from build123d import *

# Parameters (mm, degrees)
SKETCH_1_W          = 32
SKETCH_1_H          = 24
EXTRUDE_1_DEPTH     = 20
EXTRUDE_2_DEPTH     = 0.6
SKETCH_3_R          = 1.75
CUT_EXTRUDE_1_DEPTH = 34.111327367
FILLET_1_R          = 3
SKETCH_4_R          = 1.241957667
SKETCH_4_R_2        = 1.176925768
EXTRUDE_3_DEPTH     = 10
SKETCH_5_R          = 1.255951998
SKETCH_5_R_2        = 1.449746198
EXTRUDE_4_DEPTH     = 15


with BuildPart() as part:
    # 草图1 → 凸台-拉伸1 (new body)
    with BuildSketch(Plane.XY):
        Rectangle(SKETCH_1_W, SKETCH_1_H)
    extrude(amount=EXTRUDE_1_DEPTH)

    # 草图2 → 凸台-拉伸2 (add)
    with BuildSketch(Plane.XY):
        Polygon((-16, 12), (-24, 0), (-16, -12), align=None)
        Polygon((16, -12), (16, 12), (24, 0), align=None)
    extrude(amount=EXTRUDE_2_DEPTH)

    # 草图3 → 切除-拉伸1 (cut, through all)
    with BuildSketch(Plane.XY.offset(0.6)):
        with Locations((-20, 0)):
            Circle(SKETCH_3_R)
        with Locations((20, 0)):
            Circle(SKETCH_3_R)
    extrude(amount=-CUT_EXTRUDE_1_DEPTH, mode=Mode.SUBTRACT)

    # 圆角1
    fillet_1_edges = [part.edges().sort_by_distance(p)[0] for p in [
        (24, 0, 0.3),
        (-24, 0, 0.3),
    ]]
    fillet(fillet_1_edges, radius=FILLET_1_R)

    # 草图4 → 凸台-拉伸3 (add)
    with BuildSketch(Plane(origin=(0, 12, 0), x_dir=(1, 0, 0), z_dir=(0, 1, 0))):
        with Locations(Location((-8.72556125, -5.075346112, 0), (0, 0, 90))):
            Circle(SKETCH_4_R)
        with Locations(Location((7.271301042, -5.075346112, 0), (0, 0, 90))):
            Circle(SKETCH_4_R_2)
    extrude(amount=EXTRUDE_3_DEPTH)

    # 草图5 → 凸台-拉伸4 (add)
    with BuildSketch(Plane.XZ.offset(12)):
        with Locations(Location((-10.840848826, 6.265195374, 0), (0, 0, 90))):
            Circle(SKETCH_5_R)
        with Locations(Location((-0.462719157, 6.265195374, 0), (0, 0, 90))):
            Circle(SKETCH_5_R)
        with Locations(Location((7.932328409, 6.265195374, 0), (0, 0, 90))):
            Circle(SKETCH_5_R_2)
    extrude(amount=EXTRUDE_4_DEPTH)


solid = part.part
Design review of the part built by this model. Coordinates are the model's own, in mm. A direction names the side the tool comes from. Coordinates: 2 decimals unless noted, no trailing zeros. Write each loop counter-clockwise with the first axis right and the second up, starting at its lowest first coordinate (ties: lowest second). Pieces come first, ordered by that corner, then holes. Notation, with made-up numbers: (76, -27) -> (115, -27) arc R15 ccw to (115, 0) -> close; hole circle Ø5 at (-22.75, 78). An arc over 180 degrees is marked (long way). Write each question's results on one line, items separated by ' | '. Start each with the question number.
(1) Tool access review of faces 1 (the face through (-7.97, 16.93, 6.06)), 2 (the face through (8, -27, 6)), 3 (the face through (-19.4, 6.9, 0.3)), 4 (the face through (0.018, -19.395, 7.425)), 5 (the face through (18, 0, 0.6)): name each direction out of +Z, -Z, +X, -X, +Y, -Y from which nothing blocks a thin tool from reaching the whole face with its end or side.
(2) For line 1 along Y through (x, z) = (14, 10); line 2 along X through (y, z) = (-2, 15.25); line 3 along Y through (x, z) = (-20, 0.35), list the stretches that pass through material, from the lowest coordinate up. Write a range as from..to.
(3) Clearance check with flat-ended pins moving along their axes: P1, Ø6, axis at x = -18.5, y = -4, coming from the +Z side; P2, Ø1, axis at x = 12.5, z = 3.5, coming from the -Y side; P3, Ø12, axis at y = -7.5, z = 12, coming from the +X side; P4, Ø2, axis at x = 18, y = -3, coming from the +Z side. State where each tip first meets the part, or that it passes through.
(4) Take a section at D-D on y = 5.5. Write out the cut boundary in (x, z).
(5) Take a section at A-A on x = 20. Write out the cut boundary in (y, z).
(6) The part is to be moulded in two halves that separate along X. For faces 6 (the face through (19.494, -6.76, 0.296)), 7 (the face through (0, 0, 20)), 8 (the face through (6.92, 16.93, 3.95)), say which applies: pulls with the +X half, pulls with the -X half, needs draft (parallel to the pull), parting line crosses it, or undercut.
(7) Take a section at B-B on y = 0. Write out the cut boundary in (x, z), and give its area (3 significant figures).
(8) Take a section at C-C on z = 13.25. Write out the cut boundary in (x, y).
Results found:
1) face 1: +Y | face 2: +Z, -Z, +X, -X, -Y | face 3: +Z, -Z, -X, +Y | face 4: -Y | face 5: +Z, +X, +Y, -Y
2) line 1: y = -12..12 | line 2: x = -16..16 | line 3: y = -6..-1.75, 1.75..6
3) P1: stops at z = 20 | P2: stops at y = -12 | P3: stops at x = 16 | P4: stops at z = 0.6
4) outline: (-20.33, 0) -> (20.33, 0) -> (20.33, 0.6) -> (16, 0.6) -> (16, 20) -> (-16, 20) -> (-16, 0.6) -> (-20.33, 0.6) -> close
5) outline: (-6, 0) -> (-1.75, 0) -> (-1.75, 0.6) -> (-6, 0.6) -> close; (1.75, 0) -> (6, 0) -> (6, 0.6) -> (1.75, 0.6) -> close
6) face 6: pulls with the +X half | face 7: needs draft | face 8: undercut
7) outline: (-23.39, 0) -> (-21.75, 0) -> (-21.75, 0.6) -> (-23.39, 0.6) -> close; (-18.25, 0) -> (18.25, 0) -> (18.25, 0.6) -> (16, 0.6) -> (16, 20) -> (-16, 20) -> (-16, 0.6) -> (-18.25, 0.6) -> close; (21.75, 0) -> (23.39, 0) -> (23.39, 0.6) -> (21.75, 0.6) -> close | area: 645 mm2
8) outline: (-16, -12) -> (16, -12) -> (16, 12) -> (-16, 12) -> close
